Verification items for the finished model (mm, model axes). Face numbers are marked on the shaded views. A direction names the side the tool comes from. Round coordinates to 2 decimals unless told otherwise and drop trailing zeros. Loops run counter-clockwise (first coordinate to the right, second up) from the corner with the lowest first, then second, coordinate; pieces in that order, holes last. Notation, with made-up numbers: (76, 68.25) - (127, 68.25) arc R19 cw to (127, 90.25) - close; hole circle Ø10 at (14.25, 85.25). An arc over 180 degrees is marked (long way). Use a Markdown table: item, result. Add a question column.
```python
from build123d import *

# Parameters (mm, degrees)
F1_DEPTH = 50.8
F2_R     = 2.54
F3_R     = 6.35
F4_DEPTH = 25.4


with BuildPart() as f1:
    # F0 (on Front) → F1 (new body)
    with BuildSketch(Plane.XZ):
        Polygon((-152.4, 25.4), (-152.4, 0), (0, 0), (152.4, 0), (152.4, 25.4), (146.05, 25.4), (146.05, 8.89), (137.16, 8.89), (137.16, 25.4), (130.81, 25.4), (130.81, 8.89), (0, 8.89), (-130.81, 8.89), (-130.81, 25.4), (-137.16, 25.4), (-137.16, 8.89), (-146.05, 8.89), (-146.05, 25.4), align=None)
    extrude(amount=F1_DEPTH)

    # F2
    f2_edges = [f1.edges().sort_by_distance(p)[0] for p in [
        (-146.05, -25.4, 25.4),
        (-152.4, -25.4, 25.4),
        (-149.225, 0, 25.4),
        (-149.225, -50.8, 25.4),
        (-130.81, -25.4, 25.4),
        (-137.16, -25.4, 25.4),
        (-133.985, 0, 25.4),
        (-133.985, -50.8, 25.4),
        (137.16, -25.4, 25.4),
        (130.81, -25.4, 25.4),
        (133.985, 0, 25.4),
        (133.985, -50.8, 25.4),
        (152.4, -25.4, 25.4),
        (146.05, -25.4, 25.4),
        (149.225, 0, 25.4),
        (149.225, -50.8, 25.4),
    ]]
    fillet(f2_edges, radius=F2_R)

    # F3 (on face) → F4 (join)
    with BuildSketch(Plane.XY.offset(8.89)):
        with Locations((0, -25.4)):
            Circle(F3_R)
    extrude(amount=F4_DEPTH)


solid = f1.part
```
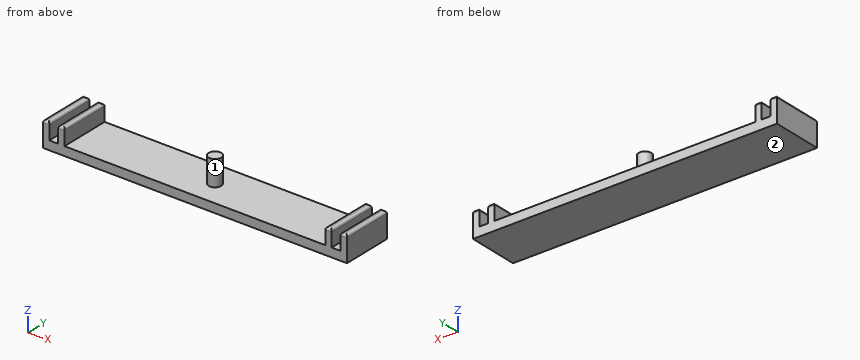
Q1. Set-up check for the marked faces 1 and 2: record each of +Z, -Z, +X, -X, +Y, -Y from which the full face is reachable in a straight line by a thin tool's end or side.
Q2. Section check A-A on z = 12.5. Record the cut outline in (x, y).
Q3. Section check B-B on y = -41.5. Record the cut outline in (x, z), plus the area to 3 significant figures.
Q4. Section check D-D on y = -25.4. Record the cut outline in (x, z), plus the area to 3 significant figures.
Q5. Section check C-C on x = 0. Record the cut outline in (y, z).
Q6. Go/stop test with flat-tipped pins: pin 1 Ø1 at (x, y) = (-134.5, -25.5) entering from +Z; pin 2 Ø10 at (x, z) = (-2, 15) entering from -Y; pin 3 Ø7 at (x, y) = (143, -30.5) entering from +Z. Record where each tip stops, or that it passes through.
Q7. Thickness scan on line 1 along X through (y, z) = (-7.5, 12); line 2 along Z through (x, y) = (112, -39); line 3 along Z through (x, y) = (-135, -34). Record the ranges inside material, lowest first.
Determined:
| question | item | result |
|---|---|---|
| 1 | face 1 | +Z |
| 1 | face 2 | -Z, +X, -X, +Y, -Y |
| 2 | outline | (-152.4, -50.8) - (-146.05, -50.8) - (-146.05, 0) - (-152.4, 0) - close; (-137.16, -50.8) - (-130.81, -50.8) - (-130.81, 0) - (-137.16, 0) - close; circle Ø12.7 at (0, -25.4); (130.81, -50.8) - (137.16, -50.8) - (137.16, 0) - (130.81, 0) - close; (146.05, -50.8) - (152.4, -50.8) - (152.4, 0) - (146.05, 0) - close |
| 3 | outline | (-152.4, 0) - (152.4, 0) - (152.4, 22.86) arc R2.54 ccw to (149.86, 25.4) - (148.59, 25.4) arc R2.54 ccw to (146.05, 22.86) - (146.05, 8.89) - (137.16, 8.89) - (137.16, 22.86) arc R2.54 ccw to (134.62, 25.4) - (133.35, 25.4) arc R2.54 ccw to (130.81, 22.86) - (130.81, 8.89) - (-130.81, 8.89) - (-130.81, 22.86) arc R2.54 ccw to (-133.35, 25.4) - (-134.62, 25.4) arc R2.54 ccw to (-137.16, 22.86) - (-137.16, 8.89) - (-146.05, 8.89) - (-146.05, 22.86) arc R2.54 ccw to (-148.59, 25.4) - (-149.86, 25.4) arc R2.54 ccw to (-152.4, 22.86) - close |
| 3 | area | 3,120 mm² |
| 4 | outline | (-152.4, 0) - (152.4, 0) - (152.4, 22.86) arc R2.54 ccw to (149.86, 25.4) - (148.59, 25.4) arc R2.54 ccw to (146.05, 22.86) - (146.05, 8.89) - (137.16, 8.89) - (137.16, 22.86) arc R2.54 ccw to (134.62, 25.4) - (133.35, 25.4) arc R2.54 ccw to (130.81, 22.86) - (130.81, 8.89) - (6.35, 8.89) - (6.35, 34.29) - (-6.35, 34.29) - (-6.35, 8.89) - (-130.81, 8.89) - (-130.81, 22.86) arc R2.54 ccw to (-133.35, 25.4) - (-134.62, 25.4) arc R2.54 ccw to (-137.16, 22.86) - (-137.16, 8.89) - (-146.05, 8.89) - (-146.05, 22.86) arc R2.54 ccw to (-148.59, 25.4) - (-149.86, 25.4) arc R2.54 ccw to (-152.4, 22.86) - close |
| 4 | area | 3,440 mm² |
| 5 | outline | (-50.8, 0) - (0, 0) - (0, 8.89) - (-19.05, 8.89) - (-19.05, 34.29) - (-31.75, 34.29) - (-31.75, 8.89) - (-50.8, 8.89) - close |
| 6 | pin 1 | stops at z = 25.4 |
| 6 | pin 2 | stops at y = -31.75 |
| 6 | pin 3 | stops at z = 24.3 |
| 7 | line 1 | x = -152.4 to -146.05, -137.16 to -130.81, 130.81 to 137.16, 146.05 to 152.4 |
| 7 | line 2 | z = 0 to 8.89 |
| 7 | line 3 | z = 0 to 25.37 |
